The figure shows three views and two pictorial views of one solid part (mm, origin at its lowest corner). Answer the questions. A direction names the side the tool comes from. Round coordinates to 2 decimals unless told otherwise and drop trailing zeros. Write each loop counter-clockwise with the first axis right and the second up, starting at its lowest first coordinate (ties: lowest second). Pieces come first, ordered by that corner, then holes.
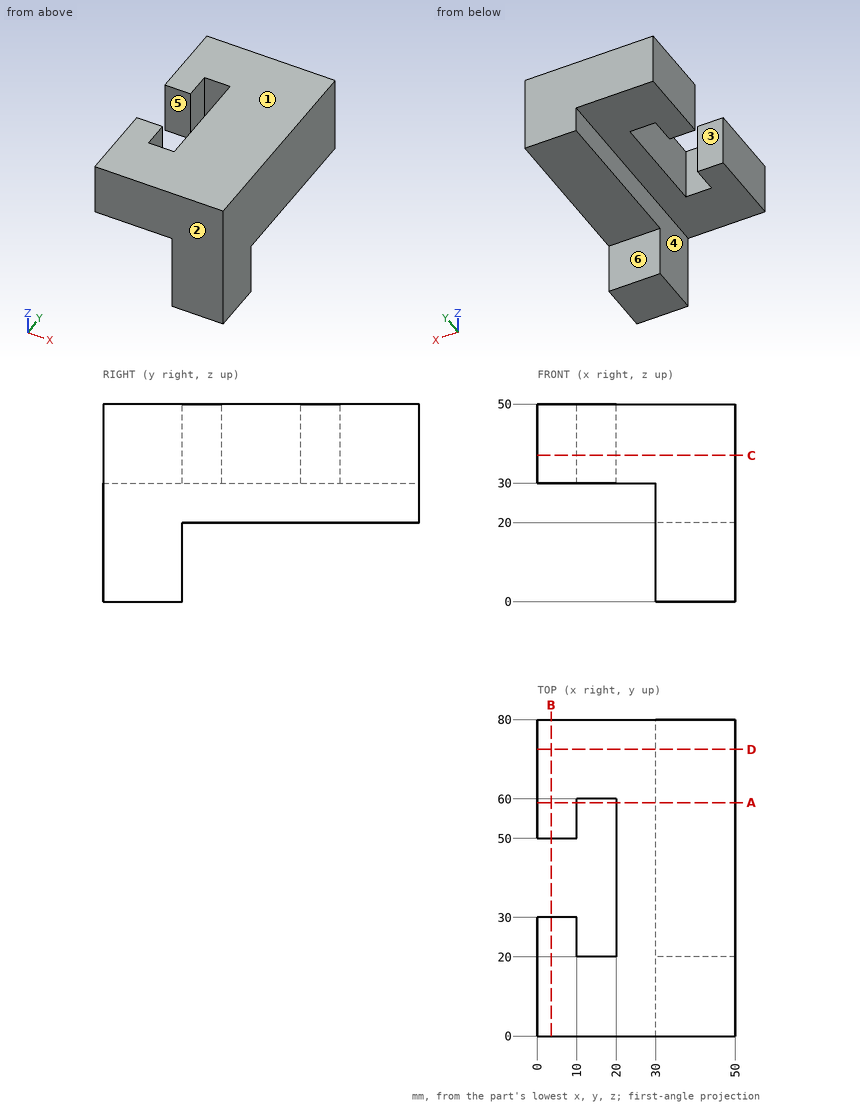
Q1. Which of the six approach directions +Z, -Z, +X, -X, +Y, -Y give full straight-line access (tool end or side, diameter ignored) to the marked faces 4, 5 and 6?
Verdict:
face 4: -Z, -X, +Y, -Y
face 5: +Z, -Z, -X
face 6: -Z, +X, -X, +Y
Q2. Section B-B (x = 3.5) is taken. Determine the outline of the cut face in (y, z), then the cut area to 3 significant figures.
Verdict:
outline: (0, 30) - (30, 30) - (30, 50) - (0, 50) - close; (50, 30) - (80, 30) - (80, 50) - (50, 50) - close
area: 1,200 mm2
Q3. Determine the mould class of the marked faces 1, 2 and 3 for opening direction Y: pulls with the +Y half, pulls with the -Y half, needs draft (parallel to the pull), parting line crosses it, or undercut.
Verdict:
face 1: needs draft
face 2: pulls with the -Y half
face 3: undercut
Q4. Straight lines are drawn through the part: probe 1 along X at (y, z) = (55.5, 34); probe 2 along Y at (x, z) = (7, 43); probe 3 along Z at (x, y) = (31, 47). For each, find the intervals that lie inside material, in ascending order.
Verdict:
probe 1: x = 0 to 10, 20 to 50
probe 2: y = 0 to 30, 50 to 80
probe 3: z = 20 to 50
Q5. Section C-C (z = 37) is taken. Determine the outline of the cut face in (x, y), then the cut area to 3 significant figures.
Verdict:
outline: (0, 0) - (50, 0) - (50, 80) - (0, 80) - (0, 50) - (10, 50) - (10, 60) - (20, 60) - (20, 20) - (10, 20) - (10, 30) - (0, 30) - close
area: 3,400 mm2
Q6. Flat-ended cylindrical pins translate along their axes: pin 1 Ø6 at (y, z) = (36, 41) entering from -X; pin 2 Ø24 at (x, y) = (14.5, 20.5) entering from -Z; pin 3 Ø8 at (y, z) = (12.5, 11.5) entering from -X. Find the tip coordinate at first contact, or state that the pin passes through.
Verdict:
pin 1: stops at x = 20
pin 2: stops at z = 30
pin 3: stops at x = 30
Q7. Section D-D (y = 72.5) is taken. Determine the outline of the cut face in (x, z), then the cut area to 3 significant figures.
Verdict:
outline: (0, 30) - (30, 30) - (30, 20) - (50, 20) - (50, 50) - (0, 50) - close
area: 1,200 mm2
Q8. Section A-A (y = 59) is taken. Determine the outline of the cut face in (x, z), then the cut area to 3 significant figures.
Verdict:
outline: (0, 30) - (10, 30) - (10, 50) - (0, 50) - close; (20, 30) - (30, 30) - (30, 20) - (50, 20) - (50, 50) - (20, 50) - close
area: 1,000 mm2
